```python
from build123d import *

# Parameters (mm, degrees)
F1_DEPTH = 40.2336
F0_R     = 10.16
F2_DEPTH = 15.7734
F3_R     = 3.302


# Not quite as in the source:
# - a feature names something its author has since deleted; it is built from what else it names


with BuildPart() as f1:
    # F0 (on Top) → F1 (new body)
    with BuildSketch(Plane.XY):
        with BuildLine():
            ThreePointArc((5.0426470588, -28.1265414802), (21.9160245563, -18.3362616868), (28.575, 0))
            ThreePointArc((28.575, 0), (21.9160245563, 18.3362616868), (5.0426470588, 28.1265414802))
            ThreePointArc((5.0426470588, 28.1265414802), (-28.575, 0), (5.0426470588, -28.1265414802))
        make_face()
        with BuildLine():
            ThreePointArc((13.4021500625, -4.9512654901), (-14.2868886671, 0.1321683185), (13.4914569997, 4.702472145))
            Line((13.4914569997, 4.702472145), (19.8402553797, 4.826))
            Line((19.8402553797, 4.826), (19.8402553797, -4.826))
            Line((19.8402553797, -4.826), (13.4021500625, -4.9512654901))
        make_face(mode=Mode.SUBTRACT)
    extrude(amount=F1_DEPTH)

    # F0 (on Top) → F2 (join)
    with BuildSketch(Plane.XY):
        with BuildLine():
            ThreePointArc((5.0426470588, 28.1265414802), (21.9160245563, 18.3362616868), (28.575, 0))
            ThreePointArc((28.575, 0), (21.9160245563, -18.3362616868), (5.0426470588, -28.1265414802))
            Line((5.0426470588, -28.1265414802), (57.3367647059, -18.7510276535))
            ThreePointArc((57.3367647059, -18.7510276535), (34.925, 0), (57.3367647059, 18.7510276535))
            Line((57.3367647059, 18.7510276535), (5.0426470588, 28.1265414802))
        make_face()
        with BuildLine():
            ThreePointArc((73.025, 0), (68.5856830375, 12.2241744579), (57.3367647059, 18.7510276535))
            ThreePointArc((57.3367647059, 18.7510276535), (34.925, 0), (57.3367647059, -18.7510276535))
            ThreePointArc((57.3367647059, -18.7510276535), (68.5856830375, -12.2241744579), (73.025, 0))
        make_face()
        with Locations((53.975, 0)):
            Circle(F0_R, mode=Mode.SUBTRACT)
    extrude(amount=F2_DEPTH)

    # F3
    f3_edges = [f1.edges().sort_by_distance(p)[0] for p in [
        (-5.042647, 28.126541, 40.2336),
    ]]
    fillet(f3_edges, radius=F3_R)


solid = f1.part
```
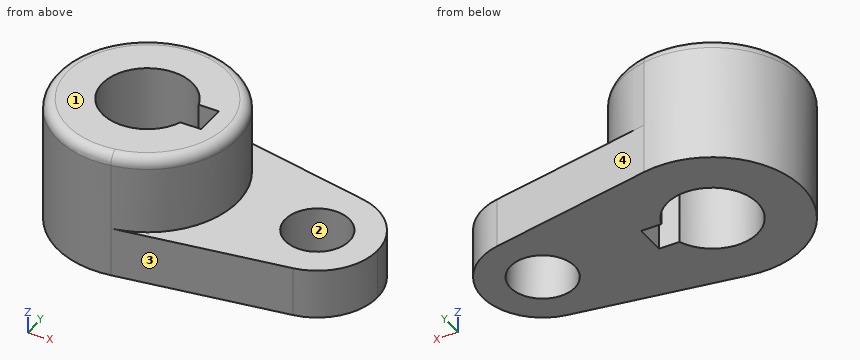
Read the model definition and answer for the solid it produces. Units are mm, in the model's axes. Face numbers are marked on the shaded views. Coordinates: 2 decimals unless noted, no trailing zeros. Write each loop counter-clockwise with the first axis right and the second up, starting at its lowest first coordinate (ties: lowest second). Pieces come first, ordered by that corner, then holes. Notation, with made-up numbers: (41.25, -36.75) - (70.25, -36.75) arc R24 ccw to (70.25, -9.75) - close; hole circle Ø8 at (0.5, 26.5). An arc over 180 degrees is marked (long way). Answer as a JSON object with one key per item and string values. Group by question number.
1. Consider L1, parallel to Y at x = 0, z = 8 (1 decimal); L2, parallel to X at y = 0, z = 27 (1 decimal); L3, parallel to X at y = -6, z = 14. Determine where each line is inside the solid, lowest interval first. Write a range as [from, to].
2. A cutting plane is placed at B-B (z = 5). Give the number of separate pieces and of enclosed holes in the cut face, plus the area to 3 significant figures.
3. Each of these flat-tipped pins is pushed along its axis until it touches: P1, Ø6, axis at x = 38, y = 21, coming from the +Z side; P2, Ø1.5, axis at y = 5, z = 34.5, coming from the +X side; P3, Ø2, axis at x = 13, z = 33, coming from the +Y side. Where does it stop, or does it pass through?
4. The mould has two halves that part along Y. Classify the marked faces 1, 2, 3 and 4: +Y half, -Y half, draft (parallel to the pull), parting line (faces both ways), or undercut.
5. A cutting plane is placed at A-A (x = 52). Determine the outline of the cut face in (y, z), plus the area to 3 significant figures.
6. A cutting plane is placed at D-D (x = 41). Determine the outline of the cut face in (y, z).
Worked out:
{
 "1": {"L1": "y = [-28.6, -14.3], [14.3, 28.6]", "L2": "x = [-28.6, -14.3], [19.8, 28.6]", "L3": "x = [-27.94, -12.97], [12.97, 45.78], [62.17, 72.06]"},
 "2": {"separate pieces": "1", "enclosed holes": "2", "area": "3,440 mm²"},
 "3": {"P1": "stops at z = 15.77", "P2": "stops at x = 28.26", "P3": "stops at y = 25.93"},
 "4": {"face 1": "draft", "face 2": "undercut", "face 3": "-Y half", "face 4": "+Y half"},
 "5": {"outline": "(-19.71, 0) - (-9.97, 0) - (-9.97, 15.77) - (-19.71, 15.77) - close; (9.97, 0) - (19.71, 0) - (19.71, 15.77) - (9.97, 15.77) - close", "area": "307 mm²"},
 "6": {"outline": "(-21.68, 0) - (21.68, 0) - (21.68, 15.77) - (-21.68, 15.77) - close"}
}
